The listing builds one solid part. Answer for the finished solid, in the listing's coordinates (mm). A direction names the side the tool comes from. Coordinates: 2 decimals unless noted, no trailing zeros. Loops run counter-clockwise (first coordinate to the right, second up) from the corner with the lowest first, then second, coordinate; pieces in that order, holes last. Notation, with made-up numbers: (36.25, 89.25) - (57.25, 89.25) arc R16 cw to (57.25, 103.25) - close; hole circle Ø3 at (81, -2). An arc over 180 degrees is marked (long way). Write each question's results on one line, items separated by ' | '. Start each with the question number.
(1) Find section A-A on y = -13. Determine the outline of the cut face in (x, z).
(2) Consider line 1 (Z direction, x = -15, y = -13.25); line 2 (Z direction, x = 4.5, y = -15.5); line 3 (X direction, y = -8, z = -3). Determine where each line is inside the solid, lowest interval first. Write a range as from..to.
(3) Given pin 1 Ø8 at (x, z) = (-17, 16.5) entering from -Y; pin 2 Ø4 at (x, z) = (-20, -21) entering from +Y, each flat-ended and moving along its own axis, determine where each tip first touches the part or whether it passes through.
(4) For faces 1 (the flat face through (0, -10, 53.84)), 2 (the flat face through (0, -10, 48.84)), determine the directions among +Z, -Z, +X, -X, +Y, -Y from which every point of the face is accessible in a straight line to the end or side of a thin tool.
(5) Determine the mould class of faces 3 (the cylindrical face through (-35.598, -10.14, 52.337)), 4 (the flat face through (0, -5, 2)), 5 (the flat face through (0, 0, 2)) for opening direction X: released by +X, released by -X, zero draft, split by the parting line, or undercut.
from build123d import *

# Parameters (mm, degrees)
F0_W     = 75
F0_H     = 105
F1_DEPTH = 20
F2_T     = -5
F3_R     = 5
F3_R_2   = 4.99999


# Not quite as in the source:
# - a fillet or chamfer is up to 0.001 mm smaller than in the source, because OpenCascade refuses the exact size


with BuildPart() as f1:
    # F0 (on Front) → F1 (new body)
    with BuildSketch(Plane.XZ):
        with Locations((0.4762494937, 1.3404280991)):
            Rectangle(F0_W, F0_H)
    extrude(amount=F1_DEPTH)

    # F2
    f2_openings = [f1.faces().sort_by_distance(p)[0] for p in [
        (0.476249, -20, 1.340428),
    ]]
    offset(amount=F2_T, openings=f2_openings)

    # F3 (call 1 of 5: OpenCascade refuses the feature's edges together)
    f3_edges = [f1.edges().sort_by_distance(p)[0] for p in [
        (-37.023751, -10, 53.840428),
    ]]
    fillet(f3_edges, radius=F3_R)

    # F3#2 (call 2 of 5)
    f3_2_edges = [f1.edges().sort_by_distance(p)[0] for p in [
        (-37.023751, -10, -51.159572),
    ]]
    fillet(f3_2_edges, radius=F3_R)

    # F3#3 (call 3 of 5)
    f3_3_edges = [f1.edges().sort_by_distance(p)[0] for p in [
        (37.976249, -10, 53.840428),
    ]]
    fillet(f3_3_edges, radius=F3_R)

    # F3#4 (call 4 of 5)
    f3_4_edges = [f1.edges().sort_by_distance(p)[0] for p in [
        (37.976249, -10, -51.159572),
    ]]
    fillet(f3_4_edges, radius=F3_R)

    # F3#5 (call 5 of 5) (radius 5 in the source; OpenCascade refuses exactly that, so slightly less here)
    f3_5_edges = [f1.edges().sort_by_distance(p)[0] for p in [
        (-32.023751, -12.5, 48.840428),
        (32.976249, -12.5, 48.840428),
        (-32.023751, -12.5, -46.159572),
        (32.976249, -12.5, -46.159572),
        (32.976249, -20, 1.340428),
        (-32.023751, -20, 1.340428),
        (0.476249, -20, 48.840428),
        (0.476249, -20, -46.159572),
    ]]
    fillet(f3_5_edges, radius=F3_R_2)


solid = f1.part
Values:
1) outline: (-37.02, -46.16) arc R5 ccw to (-32.02, -51.16) - (32.98, -51.16) arc R5 ccw to (37.98, -46.16) - (37.98, 48.84) arc R5 ccw to (32.98, 53.84) - (-32.02, 53.84) arc R5 ccw to (-37.02, 48.84) - close; hole (-32.02, -41.16) arc R5 ccw to (-27.02, -46.16) - (27.98, -46.16) arc R5 ccw to (32.98, -41.16) - (32.98, 43.84) arc R5 ccw to (27.98, 48.84) - (-27.02, 48.84) arc R5 ccw to (-32.02, 43.84) - close
2) line 1: z = -51.16..-46.16, 48.84..53.84 | line 2: z = -51.16..-46.18, 48.87..53.84 | line 3: x = -37.02..-32.02, 32.98..37.98
3) pin 1: stops at y = -5 | pin 2: stops at y = 0
4) face 1: +Z, +X, -X, +Y, -Y | face 2: -Y
5) face 3: released by -X | face 4: undercut | face 5: zero draft
